Source: CAD feature listing. Evaluate the final solid. Frame: model axes, mm. A direction names the side the tool comes from. Give positions to 0.01 mm unless a question says otherwise; leave off trailing zeros. Order: outer loops, then holes, each group sorted by start corner. A loop starts at its lowest first (then second) coordinate and runs counter-clockwise, first axis right, second up.
Autodesk Inventor part; units mm, degrees
ref_plane "YZ Plane" through (0, 0, 0) normal (1, 0, 0) x (0, 1, 0)
ref_plane "XZ Plane" through (0, 0, 0) normal (0, 1, 0) x (-1, 0, 0)
ref_plane "XY Plane" through (0, 0, 0) normal (0, 0, 1) x (1, 0, 0)
sketch "Sketch1" plane through (0, 0, 0) normal (0, 0, 1) x (1, 0, 0)
  circle A0 centre (0, 0) radius 34
  dimension "d0" = 68
extrude "Extrusion1" add sketch "Sketch1" along normal blind 98.6
sketch "Sketch2" plane through (0, 0, 0) normal (0, 1, 0) x (-1, 0, 0)
  circle A0 centre (-37, -39.4) radius 38
  line L0 (34, 98.6) -> (-34, 98.6)
  point P0 (0, 0)
  dimension "d3" = 76
  dimension "d4" = 138
  dimension "d5" = 37
extrude "Extrusion2" add sketch "Sketch2" along normal blind 90.5 and the other way blind 20
sketch "Sketch3" plane through (37, 90.5, -39.4) normal (0, 1, 0) x (1, 0, 0)
  circle A0 centre (0, 0) radius 53
  circle A1 centre (0, 0) radius 38
  point P0 (-37, -39.4)
  dimension "d10" = 106
extrude "Extrusion3" add sketch "Sketch3" against normal blind 3
sketch "Sketch4" plane through (0, 0, 0) normal (0, 1, 0) x (-1, 0, 0)
  circle A0 centre (-37, -39.4) radius 38
  line L0 (0, 0) -> (-37, 0)
  line L1 (-34, 0) -> (34, 0)
  line L2 (0, 0) -> (0, -39.4)
  line L3 (0, -39.4) -> (-37, -39.4)
  line L4 (-37, -39.4) -> (-37, 0)
extrude "Extrusion4" add sketch "Sketch4" along normal blind 10 and the other way blind 20 contours L2 L3 L4 A0 | A0 L4 L0 L2 picked at (-12.3333, -36.5132)
sketch "Sketch5" plane through (37, 90.5, -39.4) normal (0, 1, 0) x (1, 0, 0)
  circle A0 centre (0, 0) radius 53 construction
  circle A1 centre (0, 0) radius 7.5
  point P0 (-37, -39.4)
  dimension "d17" = 15
extrude "Extrusion5" add sketch "Sketch5" along normal blind 50
sketch "Sketch6" plane through (37, 90.5, -39.4) normal (0, 1, 0) x (1, 0, 0)
  circle A0 centre (0, 0) radius 53 construction
  circle A1 centre (23.5, 40.7032) radius 3.1
  line L0 (0, 0) -> (0, 53) construction
  line L1 (0, 0) -> (23.5, 40.7032) construction
  circle A2 centre (-47, 0) radius 3.1
  circle A3 centre (23.5, -40.7032) radius 3.1
  circle A4 centre (0, 47) radius 3.1
  circle A5 centre (-47, 0) radius 3.1
  circle A6 centre (0, -47) radius 3.1
  circle A7 centre (47, 0) radius 3.1
  point P0 (-37, -39.4)
  dimension "d20" = 6.2
  dimension "d21" = 47
  dimension "d22" = 30
  dimension "d25" = 360
  dimension "d27" = 6.2
  dimension "d28" = 47
  dimension "d31" = 360
extrude "Extrusion6" cut sketch "Sketch6" against normal through all
properties part number "PN00113-6" material "ABS Plastic"
1) Section query C-C, the plane y = 0. Return the cut outline in (x, z).
Report:
outline: (-34, 0) - (0, 0) - (0, -30.74) arc R38 ccw (long way) to (37, -1.4) - (37, 0) - (34, 0) - (34, 6.82) arc R3.1 cw to (34, 8.38) - (34, 98.6) - (-34, 98.6) - close
2) Section query A-A, the plane z = -39.4. Return the cut outline in (x, y), and give its area (3 significant figures).
Report:
outline: (-16, 87.5) - (-13.1, 87.5) - (-13.1, 90.5) - (-16, 90.5) - close; (-6.9, 87.5) - (-1, 87.5) - (-1, -20) - (75, -20) - (75, 87.5) - (80.9, 87.5) - (80.9, 90.5) - (44.5, 90.5) - (44.5, 140.5) - (29.5, 140.5) - (29.5, 90.5) - (-6.9, 90.5) - close; (87.1, 87.5) - (90, 87.5) - (90, 90.5) - (87.1, 90.5) - close
area: 9,200 mm2
3) Reachability of faces 1 (the flat face through (0, -5, -15)), 2 (the flat face through (38, -20, -38)), 3 (the flat face through (10, 10, -7)) from +Z, -Z, +X, -X, +Y, -Y: full face, straight path, thin tool, end or side. Return the list, or none.
Report:
face 1: -X, -Y
face 2: -Z, +X, -X, -Y
face 3: -X
4) Section query D-D, the plane z = -7. Return the cut outline in (x, y), and give its area (3 significant figures).
Report:
outline: (-4.94, 87.5) - (17.14, 87.5) - (17.14, 10) - (0, 10) - (0, -20) - (56.86, -20) - (56.86, 87.5) - (78.94, 87.5) - (78.94, 90.5) - (-4.94, 90.5) - close
area: 5,030 mm2
5) Material intervals for L1, parallel to X at y = 88, z = -39; L2, parallel to Z at x = 37, y = 89; L3, parallel to Y at x = 24, z = -40, sorted ascending.
Report:
L1: x = -16 to -13.07, -6.93 to 80.93, 87.07 to 90
L2: z = -92.4 to -89.5, -83.3 to 4.5, 10.7 to 13.6
L3: y = -20 to 90.5
6) Section query B-B, the plane x = 53. Return the cut outline in (y, z).
Report:
outline: (-20, -73.87) - (87.5, -73.87) - (87.5, -89.93) - (90.5, -89.93) - (90.5, 11.13) - (87.5, 11.13) - (87.5, -4.93) - (-20, -4.93) - close
7) Pin query (flat end, axial travel): pin 1 (7 mm diameter, centred on x = 60.5, z = 1.3, fed in from +Y); pin 2 (4 mm diameter, centred on y = 30.5, z = 3.5, fed in from -X); pin 3 (9 mm diameter, centred on y = -1, z = -14, fed in from -X). Return the tip coordinate at first contact, or that it passes through.
Report:
pin 1: stops at y = 90.5
pin 2: stops at x = -18.54
pin 3: stops at x = 0
8) Draft query along Y for faces 4 (the flat face through (37, 140.5, -40)), 5 (the cylindrical face through (65.01, 33, -65.08)), 6 (the cylindrical face through (39.864, 89.021, 8.787)). Return one class per face: +Y half, -Y half, draft (parallel to the pull), parting line (faces both ways), or undercut.
Report:
face 4: +Y half
face 5: undercut
face 6: draft
